```python
from build123d import *

# Parameters (mm, degrees)
SKETCH1_W                                    = 114.3
SKETCH1_H                                    = 63.5
BOSS_EXTRUDE3_DEPTH                          = 12.7
FILLET1_R                                    = 5.08
CBORE_FOR_1_4_HEX_MACHINE_SCREW1_D           = 6.7564
CBORE_FOR_1_4_HEX_MACHINE_SCREW1_CBORE_D     = 15.875
CBORE_FOR_1_4_HEX_MACHINE_SCREW1_CBORE_DEPTH = 4.826


with BuildPart() as part:
    # Sketch1 → Boss-Extrude3 (new body)
    with BuildSketch(Plane.XY):
        with BuildLine():
            ThreePointArc((-139.7, 0), (-98.782817332, 98.782817332), (0, 139.7))
            Line((0, 139.7), (0, 495.3))
            Line((0, 495.3), (-203.2, 495.3))
            Line((-203.2, 495.3), (-254, 165.1))
            Line((-254, 165.1), (-254, 0))
            Line((-254, 0), (-139.7, 0))
        make_face()
        with Locations((-196.85, -31.75)):
            Rectangle(SKETCH1_W, SKETCH1_H)
        with BuildLine():
            ThreePointArc((0, 139.7), (98.782817332, 98.782817332), (139.7, 0))
            Line((139.7, 0), (254, 0))
            Line((254, 0), (254, 165.1))
            Line((254, 165.1), (203.2, 495.3))
            Line((203.2, 495.3), (0, 495.3))
            Line((0, 495.3), (0, 139.7))
        make_face()
        with Locations((196.85, -31.75)):
            Rectangle(SKETCH1_W, SKETCH1_H)
    extrude(amount=BOSS_EXTRUDE3_DEPTH)

    # Fillet1
    fillet1_edges = [part.edges().sort_by_distance(p)[0] for p in [
        (-139.7, -63.5, 6.35),
        (-254, -63.5, 6.35),
        (-254, 165.1, 6.35),
        (-203.2, 495.3, 6.35),
        (203.2, 495.3, 6.35),
        (254, 165.1, 6.35),
        (254, -63.5, 6.35),
        (139.7, -63.5, 6.35),
    ]]
    fillet(fillet1_edges, radius=FILLET1_R)

    # CBORE for 1/4 Hex Machine Screw1 (through all)
    with Locations(Plane.XY.offset(12.7)):
        with Locations((165.1, 482.6), (165.1, 152.4), (-165.1, 152.4), (-165.1, 482.6)):
            CounterBoreHole(CBORE_FOR_1_4_HEX_MACHINE_SCREW1_D / 2, CBORE_FOR_1_4_HEX_MACHINE_SCREW1_CBORE_D / 2, CBORE_FOR_1_4_HEX_MACHINE_SCREW1_CBORE_DEPTH)


solid = part.part
```
Verification items for the finished model (mm, model axes). A direction names the side the tool comes from. Coordinates: 2 decimals unless noted, no trailing zeros. Loops run counter-clockwise (first coordinate to the right, second up) from the corner with the lowest first, then second, coordinate; pieces in that order, holes last. Notation, with made-up numbers: (83.25, -28.75) -> (124.25, -28.75) arc R18 cw to (124.25, 1.25) -> close; hole circle Ø11 at (2.5, 46). An arc over 180 degrees is marked (long way). Answer in a Markdown table with one row per item.
1) Draft check along X on faces 1 (the face through (-228.55, 330.52, 6.26)), 2 (the face through (-163, 149, 7.874)), 3 (the face through (254, 52, 6)). Enter one of: released by +X, released by -X, zero draft, split by the parting line, or undercut.
The answers:
| item | result |
|---|---|
| face 1 | released by -X |
| face 2 | undercut |
| face 3 | released by +X |
2) Section check C-C (x = -51). Record the cut outline in (y, z), and give its area (3 significant figures).
The answers:
| item | result |
|---|---|
| outline | (130.06, 0) -> (495.3, 0) -> (495.3, 12.7) -> (130.06, 12.7) -> close |
| area | 4,640 mm2 |
3) Section check A-A (z = 2.5). Record the cut outline in (x, y).
The answers:
| item | result |
|---|---|
| outline | (-254, -58.42) arc R5.08 ccw to (-248.92, -63.5) -> (-144.78, -63.5) arc R5.08 ccw to (-139.7, -58.42) -> (-139.7, 0) arc R139.7 cw to (139.7, 0) -> (139.7, -58.42) arc R5.08 ccw to (144.78, -63.5) -> (248.92, -63.5) arc R5.08 ccw to (254, -58.42) -> (254, 164.71) arc R5.08 ccw to (253.94, 165.48) -> (203.86, 490.99) arc R5.08 ccw to (198.84, 495.3) -> (-198.84, 495.3) arc R5.08 ccw to (-203.86, 490.99) -> (-253.94, 165.48) arc R5.08 ccw to (-254, 164.71) -> close; hole circle Ø6.76 at (-165.1, 152.4); hole circle Ø6.76 at (-165.1, 482.6); hole circle Ø6.76 at (165.1, 152.4); hole circle Ø6.76 at (165.1, 482.6) |
4) Section check D-D (y = 394). Record the cut outline in (x, z).
The answers:
| item | result |
|---|---|
| outline | (-218.78, 0) -> (218.78, 0) -> (218.78, 12.7) -> (-218.78, 12.7) -> close |
5) Scan lines: line 1 along Y through (x, z) = (165.1, 11.6); line 2 along Y through (x, z) = (165.1, 1.5); line 3 along X through (y, z) = (482.6, 5). Record each from-to range of solid material in increasing order. Write a range as from..to.
The answers:
| item | result |
|---|---|
| line 1 | y = -63.5..144.46, 160.34..474.66, 490.54..495.3 |
| line 2 | y = -63.5..149.02, 155.78..479.22, 485.98..495.3 |
| line 3 | x = -205.15..-168.48, -161.72..161.72, 168.48..205.15 |
6) Depth check by flat-ended pin: P1, Ø12.5, axis at x = 165.1, y = 152.4, coming from the +Z side; P2, Ø1.5, axis at y = 312.5, z = 2.5, coming from the -X side. Enter the tip coordinate at first touch or a pass-through.
The answers:
| item | result |
|---|---|
| P1 | stops at z = 7.87 |
| P2 | stops at x = -231.44 |
7) Access from +Z, -Z, +X, -X, +Y, -Y to the whole of each face (thin tool, end or side, straight path). Record for faces 4 (the face through (-157.529, 154.784, 10.321)), 5 (the face through (-139.7, -30, 6)), 6 (the face through (196, -63.5, 6)).
The answers:
| item | result |
|---|---|
| face 4 | +Z |
| face 5 | +Z, -Z, -Y |
| face 6 | +Z, -Z, +X, -X, -Y |
8) Section check B-B (y = 39). Record the cut outline in (x, z), and give its area (3 significant figures).
The answers:
| item | result |
|---|---|
| outline | (-254, 0) -> (-134.15, 0) -> (-134.15, 12.7) -> (-254, 12.7) -> close; (134.15, 0) -> (254, 0) -> (254, 12.7) -> (134.15, 12.7) -> close |
| area | 3,040 mm2 |
